Input: part model. Units: mm. Frame: model coordinates. A direction names the side the tool comes from. Coordinates: 2 decimals unless noted, no trailing zeros. Write each loop counter-clockwise with the first axis right and the second up, starting at its lowest first coordinate (ties: lowest second). Pieces come first, ordered by that corner, then holes. Notation, with made-up numbers: M -17.5,-23.75 L 15.5,-23.75 A9 ccw 15.5,-11.75 Z; hole C -19.75,68.5 d1. An arc over 180 degrees is marked long. Use CSV: the item, a comma, the result in double quotes.
```python
from build123d import *

# Parameters (mm, degrees)
SKETCH1_W           = 2.54
SKETCH1_H           = 31.75
BOSS_EXTRUDE1_DEPTH = 49.9999
SKETCH5_R           = 2.99974
SKETCH5_R_2         = 1.6002
BOSS_EXTRUDE3_DEPTH = 8.6106


with BuildPart() as part:
    # Sketch1 → Boss-Extrude1 (new body)
    with BuildSketch(Plane(origin=(0, 0, 0), x_dir=(1, 0, 0), z_dir=(0, 1, 0))):
        with Locations((1.27, 15.875)):
            Rectangle(SKETCH1_W, SKETCH1_H)
    extrude(amount=BOSS_EXTRUDE1_DEPTH)

    # Sketch5 → Boss-Extrude3 (add)
    with BuildSketch(Plane(origin=(0, 0, 0), x_dir=(0, 0, -1), z_dir=(1, 0, 0))):
        with Locations((15.875, 15.00124)):
            Circle(SKETCH5_R)
        with Locations((15.875, 15.00124)):
            Circle(SKETCH5_R_2, mode=Mode.SUBTRACT)
        with Locations((15.875, 35.0012)):
            Circle(SKETCH5_R)
        with Locations((15.875, 35.0012)):
            Circle(SKETCH5_R_2, mode=Mode.SUBTRACT)
    extrude(amount=-BOSS_EXTRUDE3_DEPTH)


solid = part.part
```
1. Material intervals for line 1 (X direction, y = 41.5, z = -28.5); line 2 (Z direction, x = -7.25, y = 34.5); line 3 (Y direction, x = -1.5, z = -13.5), sorted ascending. Write a range as [from, to].
Resolved:
line 1,"x = [0, 2.54]"
line 2,"z = [-18.83, -17.39], [-14.36, -12.92]"
line 3,"y = [13.17, 16.83], [33.17, 36.83]"
2. Section A-A (x = -6.75). Return loops of the section in (y, z) (3 decimals).
Resolved:
outline,"C 15.001,-15.875 d5.999; C 35.001,-15.875 d5.999; hole C 15.001,-15.875 d3.2; hole C 35.001,-15.875 d3.2"
3. Access query for faces 1 (the flat face through (-8.611, 13.7, -17.2)), 2 (the cylindrical face through (-4.25, 35.48, -17.4)). Directions: +Z, -Z, +X, -X, +Y, -Y. A direction counts if a zero-diameter tool reaches every point of the face in a straight line with its end or side. Return the directions, or none.
Resolved:
face 1,"+Z, -Z, -X, +Y, -Y"
face 2,"-X"
4. Section C-C (y = 25.5). Return loops of the section in (x, z), then the cut area to 3 significant figures.
Resolved:
outline,"M 0,-31.75 L 2.54,-31.75 L 2.54,0 L 0,0 Z"
area,"80.6 mm^2"
5. Section B-B (z = -11.5). Return loops of the section in (x, y), then the cut area to 3 significant figures.
Resolved:
outline,"M 0,0 L 2.54,0 L 2.54,50 L 0,50 Z"
area,"127 mm^2"
6. Contact query for flat-ended pins moving along their axis: pin 1 Ø2.5 at (y, z) = (35.5, -16.5) entering from -X; pin 2 Ø4 at (x, z) = (-3.5, -16) entering from -Y; pin 3 Ø2 at (x, z) = (-4.5, -12.5) entering from -Y; pin 4 Ø6 at (y, z) = (7.5, -13.5) entering from -X. Output: stop coordinate, or through.
Resolved:
pin 1,"stops at x = -8.61"
pin 2,"stops at y = 12"
pin 3,"stops at y = 13.17"
pin 4,"stops at x = 0"
7. Mould query, pull axis Z, two halves, no side actions, for faces 3 (the cylindrical face through (-4.25, 17.53, -17.49)), 4 (the flat face through (0, 25, -16)), 5 (the flat face through (0, 35, -16)). Classes: pulls with the +Z half, pulls with the -Z half, needs draft (parallel to the pull), parting line crosses it, or undercut.
Resolved:
face 3,"parting line crosses it"
face 4,"needs draft"
face 5,"undercut"
